from build123d import *

# Parameters (mm, degrees)
F0_W     = 2438.4
F0_H     = 1219.2
F1_DEPTH = 457.2
F2_W     = 457.2
F2_H     = 127
F3_DEPTH = 457.2


with BuildPart() as f1:
    # F0 (on Front) → F1 (new body, symmetric)
    with BuildSketch(Plane.XZ):
        Rectangle(F0_W, F0_H)
    extrude(amount=F1_DEPTH, both=True)

    # F2 (on face) → F3 (cut)
    with BuildSketch(Plane.XY.offset(609.6)):
        with Locations((-965.2, 368.3)):
            Rectangle(F2_W, F2_H)
        with Locations((-962.697564, 215.920547)):
            Rectangle(F2_W, F2_H)
        with Locations((-960.195127, 63.541093)):
            Rectangle(F2_W, F2_H)
        with Locations((-957.692691, -88.83836)):
            Rectangle(F2_W, F2_H)
        with Locations((-955.190254, -241.217814)):
            Rectangle(F2_W, F2_H)
        with Locations((-482.607881, 365.542049)):
            Rectangle(F2_W, F2_H)
        with Locations((-480.105444, 213.162596)):
            Rectangle(F2_W, F2_H)
        with Locations((-477.603008, 60.783143)):
            Rectangle(F2_W, F2_H)
        with Locations((-475.100571, -91.596311)):
            Rectangle(F2_W, F2_H)
        with Locations((-472.598135, -243.975764)):
            Rectangle(F2_W, F2_H)
        with Locations((-0.015761, 362.784099)):
            Rectangle(F2_W, F2_H)
        with Locations((2.486675, 210.404645)):
            Rectangle(F2_W, F2_H)
        with Locations((4.989112, 58.025192)):
            Rectangle(F2_W, F2_H)
        with Locations((7.491548, -94.354261)):
            Rectangle(F2_W, F2_H)
        with Locations((9.993984, -246.733715)):
            Rectangle(F2_W, F2_H)
        with Locations((482.576358, 360.026148)):
            Rectangle(F2_W, F2_H)
        with Locations((485.078795, 207.646695)):
            Rectangle(F2_W, F2_H)
        with Locations((487.581231, 55.267242)):
            Rectangle(F2_W, F2_H)
        with Locations((490.083667, -97.112212)):
            Rectangle(F2_W, F2_H)
        with Locations((492.586104, -249.491665)):
            Rectangle(F2_W, F2_H)
        with Locations((965.168478, 357.268198)):
            Rectangle(F2_W, F2_H)
        with Locations((967.670914, 204.888744)):
            Rectangle(F2_W, F2_H)
        with Locations((970.17335, 52.509291)):
            Rectangle(F2_W, F2_H)
        with Locations((972.675787, -99.870162)):
            Rectangle(F2_W, F2_H)
        with Locations((975.178223, -252.249616)):
            Rectangle(F2_W, F2_H)
    extrude(amount=-F3_DEPTH, mode=Mode.SUBTRACT)


solid = f1.part
For this review, take the finished solid that the model builds, in its own axes (mm). Coordinates: 2 decimals unless noted, no trailing zeros. Loops run counter-clockwise (first coordinate to the right, second up) from the corner with the lowest first, then second, coordinate; pieces in that order, holes last. Notation, with made-up numbers: (-21.75, 3.25) - (-15.75, 3.25) arc R14 ccw to (-15.75, 24.25) - close; hole circle Ø8 at (-18.75, 40). An arc over 180 degrees is marked (long way). Use a Markdown table: item, result. Add a question column.
Item 1: We need section A-A (x = -450.5). Give the boundary of the cut face in (y, z).
Item 2: For line 1 (X direction, y = 363.5, z = 484); line 2 (X direction, y = -183, z = 249.5); line 3 (Z direction, x = 134.5, y = 309), list the stretches that pass through material, from the lowest coordinate up.
Item 3: We need section C-C (z = 518). Give the number of separate pieces and of enclosed holes in the cut face, and give its area (3 significant figures).
Item 4: We need section B-B (y = 42). Give the boundary of the cut face in (x, z), and give its area (3 significant figures).
Results list:
| question | item | result |
|---|---|---|
| 1 | outline | (-457.2, -609.6) - (457.2, -609.6) - (457.2, 609.6) - (429.04, 609.6) - (429.04, 152.4) - (302.04, 152.4) - (302.04, 609.6) - (276.66, 609.6) - (276.66, 152.4) - (149.66, 152.4) - (149.66, 609.6) - (124.28, 609.6) - (124.28, 152.4) - (-2.72, 152.4) - (-2.72, 609.6) - (-28.1, 609.6) - (-28.1, 152.4) - (-155.1, 152.4) - (-155.1, 609.6) - (-180.48, 609.6) - (-180.48, 152.4) - (-307.48, 152.4) - (-307.48, 609.6) - (-457.2, 609.6) - close |
| 2 | line 1 | x = -1219.2 to -1193.8, -736.6 to -711.21, -254.01 to -228.62, 228.58 to 253.98, 711.18 to 736.57, 1193.77 to 1219.2 |
| 2 | line 2 | x = -1219.2 to -1183.79, -726.59 to -701.2, -244 to 1219.2 |
| 2 | line 3 | z = -609.6 to 152.4 |
| 3 | separate pieces | 1 |
| 3 | enclosed holes | 25 |
| 3 | area | 778,000 mm^2 |
| 4 | outline | (-1219.2, -609.6) - (1219.2, -609.6) - (1219.2, 609.6) - (1198.77, 609.6) - (1198.77, 152.4) - (741.57, 152.4) - (741.57, 609.6) - (716.18, 609.6) - (716.18, 152.4) - (258.98, 152.4) - (258.98, 609.6) - (233.59, 609.6) - (233.59, 152.4) - (-223.61, 152.4) - (-223.61, 609.6) - (-249, 609.6) - (-249, 152.4) - (-706.2, 152.4) - (-706.2, 609.6) - (-731.6, 609.6) - (-731.6, 152.4) - (-1188.8, 152.4) - (-1188.8, 609.6) - (-1219.2, 609.6) - close |
| 4 | area | 1,930,000 mm^2 |
